Geometry: final body of the model. Coordinates: model frame, mm. A direction names the side the tool comes from. Round coordinates to 2 decimals unless told otherwise and drop trailing zeros. Loops run counter-clockwise (first coordinate to the right, second up) from the corner with the lowest first, then second, coordinate; pieces in that order, holes last. Notation, with made-up numbers: (68.25, 47) - (97.25, 47) arc R29 cw to (97.25, 77) - close; hole circle Ø5 at (32, 44.25). An arc over 180 degrees is marked (long way). Answer in a Markdown table with one row per item. Add a question column.
from build123d import *
from build123d.topology import SkipClean

# Parameters (mm, degrees)
SKETCH1_R               = 5.6
SKETCH1_R_2             = 1.6
BOSS_EXTRUDE1_DEPTH     = 10
SKETCH2_R               = 5.6
BOSS_EXTRUDE2_DEPTH     = 2
BOSS_EXTRUDE3_DEPTH     = 10
CUT_EXTRUDE1_DEPTH      = 25.004166
CUT_EXTRUDE1_DEPTH_BACK = 25.004166
SKETCH4_R               = 1.75
FILLET1_SIZE            = 10
FILLET1_SIZE_2          = 3


with BuildPart() as part:
    # Sketch1 → Boss-Extrude1 (new body)
    with BuildSketch(Plane(origin=(0, 0, 0), x_dir=(1, 0, 0), z_dir=(0, 1, 0))):
        with Locations(Location((0, 0, 0), (0, 0, 270))):
            Circle(SKETCH1_R)
        with Locations(Location((0, 0, 0), (0, 0, 270))):
            Circle(SKETCH1_R_2, mode=Mode.SUBTRACT)
    extrude(amount=BOSS_EXTRUDE1_DEPTH)

    # Sketch2 → Boss-Extrude2 (add)
    with BuildSketch(Plane(origin=(0, 10, 0), x_dir=(1, 0, 0), z_dir=(0, 1, 0))):
        with Locations(Location((0, 0, 0), (0, 0, 270))):
            Circle(SKETCH2_R)
    extrude(amount=BOSS_EXTRUDE2_DEPTH)

    # Sketch3 → Boss-Extrude3 (add)
    with BuildSketch(Plane(origin=(0, 12, 0), x_dir=(1, 0, 0), z_dir=(0, 1, 0))):
        with BuildLine():
            Line((-5.149757, 2.2), (5.149757, 2.2))
            ThreePointArc((5.149757, 2.2), (0, 5.6), (-5.149757, 2.2))
        make_face()
        with BuildLine():
            Line((-5.149757, -2.2), (5.149757, -2.2))
            ThreePointArc((5.149757, -2.2), (0, -5.6), (-5.149757, -2.2))
        make_face()
    extrude(amount=BOSS_EXTRUDE3_DEPTH)

    # Sketch4 → Cut-Extrude1 (cut, two sides: drawn at the far end of the back side and taken through both)
    with SkipClean():  # the faces are left unmerged after this step: merging them gives an invalid solid
        with BuildSketch(Plane(origin=(0, 0, 2.2), x_dir=(-1, 0, 0), z_dir=(0, 0, -1)).offset(-CUT_EXTRUDE1_DEPTH_BACK)):
            with BuildLine():
                Line((5.149757, 22.1), (5.149757, 22))
                Line((5.149757, 22), (1.232883, 22))
                ThreePointArc((1.232883, 22), (4.053952, 20.175764), (5.149757, 17))
                Line((5.149757, 17), (5.149757, 12))
                Line((5.149757, 12), (5.249757, 12))
                Line((5.249757, 12), (5.249757, 22.1))
                Line((5.249757, 22.1), (5.149757, 22.1))
            make_face()
            with BuildLine():
                ThreePointArc((-5.149757, 17), (-4.053952, 20.175764), (-1.232883, 22))
                Line((-1.232883, 22), (-5.149757, 22))
                Line((-5.149757, 22), (-5.149757, 22.1))
                Line((-5.149757, 22.1), (-5.249757, 22.1))
                Line((-5.249757, 22.1), (-5.249757, 12))
                Line((-5.249757, 12), (-5.149757, 12))
                Line((-5.149757, 12), (-5.149757, 17))
            make_face()
            with Locations(Location((0, 17, 0), (0, 0, 270))):
                Circle(SKETCH4_R)
        extrude(amount=CUT_EXTRUDE1_DEPTH + CUT_EXTRUDE1_DEPTH_BACK, mode=Mode.SUBTRACT)

    # Fillet1
    # an asymmetric fillet: 10, 3 mm, written as the material it takes off along each edge
    with BuildSketch(Plane(origin=(0, 0, 0), x_dir=(0, 0, 1), z_dir=(-1, 0, 0))) as fillet1_piece_1:
        with BuildLine():
            Bezier((5.6, FILLET1_SIZE), (5.6, 0), (5.6 - FILLET1_SIZE_2, 0), weights=[1, 0.707107, 1])
            Line((5.6 - FILLET1_SIZE_2, 0), (5.6, 0))
            Line((5.6, 0), (5.6, FILLET1_SIZE))
        make_face()
    revolve(axis=Axis((0, 0, 0), (0, 1, 0)), mode=Mode.SUBTRACT)


solid = part.part
1) Material intervals for line 1 along Y through (x, z) = (-3.75, 1.5); line 2 along Y through (x, z) = (0, -0.5); line 3 along X through (y, z) = (18.5, 3), sorted ascending. Write a range as from..to.
2) Pull-direction query (X, two-part tool) for faces 4 (the cylindrical face through (-2.91, 21.25, 3.49)), 5 (the cylindrical face through (2.993, 21.191, 3.492)), 6 (the flat face through (0, 22, -4)), 7 (the cylindrical face through (-0.97, 4.93, -1.27)); classes: pulls with the +X half, pulls with the -X half, needs draft (parallel to the pull), parting line crosses it, or undercut.
3) Contact query for flat-ended pins moving along their axis: pin 1 Ø1.5 at (x, y) = (-1.5, 17.5) entering from -Z; pin 2 Ø2 at (x, y) = (0, 17) entering from +Z; pin 3 Ø1 at (y, z) = (10, 3) entering from +X; pin 4 Ø3 at (x, z) = (0, 0) entering from -Y. Output: stop coordinate, or through.
4) Section B-B, the plane y = 20.25. Return the cut outline in (x, z), and give its area (3 significant figures).
5) Section A-A, the plane y = 17.25. Give the number of separate pieces and of enclosed holes in the cut face, and give its area (3 significant figures).
6) Reachability of faces 1 (the flat face through (0, 15, -2.2)), 2 (the cylindrical face through (-1.735, 17.228, -3.879)), 3 (the flat face through (0, 10, 0)) from +Z, -Z, +X, -X, +Y, -Y: full face, straight path, thin tool, end or side. Return the list, or none.
Evaluation:
| question | item | result |
|---|---|---|
| 1 | line 1 | y = 1.23..12 |
| 1 | line 2 | y = 10..12 |
| 1 | line 3 | x = -4.73..-0.9, 0.9..4.73 |
| 2 | face 4 | pulls with the -X half |
| 2 | face 5 | pulls with the +X half |
| 2 | face 6 | needs draft |
| 2 | face 7 | undercut |
| 3 | pin 1 | stops at z = -5.46 |
| 3 | pin 2 | passes through |
| 3 | pin 3 | stops at x = 5.01 |
| 3 | pin 4 | stops at y = 10 |
| 4 | outline | (-3.99, -3.92) arc R5.6 ccw to (3.99, -3.92) - (3.99, -2.2) - (-3.99, -2.2) - close; (-3.99, 2.2) - (3.99, 2.2) - (3.99, 3.92) arc R5.6 ccw to (-3.99, 3.92) - close |
| 4 | area | 46.0 mm² |
| 5 | separate pieces | 4 |
| 5 | enclosed holes | 0 |
| 5 | area | 27.6 mm² |
| 6 | face 1 | +X, -X, +Y |
| 6 | face 2 | +Z, -Z |
| 6 | face 3 | -Y |
